```python
from build123d import *

# Parameters (mm, degrees)
SKETCH_1_W      = 90.450741223
SKETCH_1_H      = 43.255156446
EXTRUDE_1_DEPTH = 10
EXTRUDE_2_DEPTH = 20
EXTRUDE_3_DEPTH = 10


with BuildPart() as part:
    # 草图1 → 凸台-拉伸1 (new body)
    with BuildSketch(Plane(origin=(0, 0, 0), x_dir=(1, 0, 0), z_dir=(0, 1, 0))):
        with Locations((45.225370612, 21.627578223)):
            Rectangle(SKETCH_1_W, SKETCH_1_H)
    extrude(amount=EXTRUDE_1_DEPTH)

    # 草图2 → 凸台-拉伸2 (add)
    with BuildSketch(Plane(origin=(0, 10, 0), x_dir=(1, 0, 0), z_dir=(0, 1, 0))):
        with BuildLine():
            Line((68.630258788, 43.255156446), (21.047365446, 43.255156446))
            ThreePointArc((21.047365446, 43.255156446), (44.838812117, 19.463709775), (68.630258788, 43.255156446))
        make_face()
    extrude(amount=EXTRUDE_2_DEPTH)

    # 草图3 → 凸台-拉伸3 (add)
    with BuildSketch(Plane.XZ):
        with BuildLine():
            Line((22.99825717, -8.71008186), (70.802657673, -8.71008186))
            ThreePointArc((70.802657673, -8.71008186), (82.399412512, -20.3068367), (70.802657673, -31.903591539))
            Line((70.802657673, -31.903591539), (22.99825717, -31.903591539))
            ThreePointArc((22.99825717, -31.903591539), (11.40150233, -20.3068367), (22.99825717, -8.71008186))
        make_face()
    extrude(amount=EXTRUDE_3_DEPTH)


solid = part.part
```
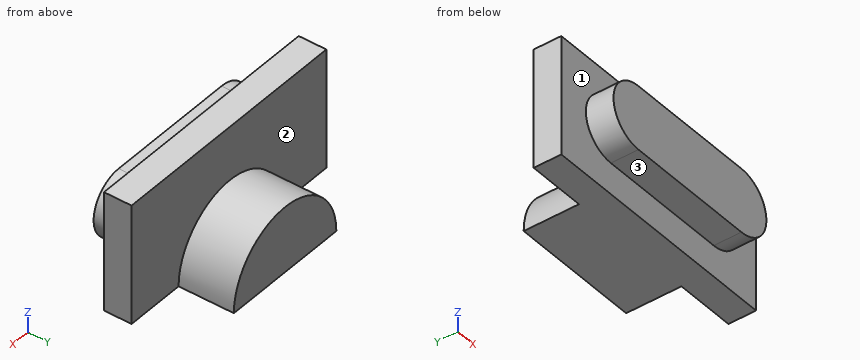
Read the model definition and answer for the solid it produces. Units are mm, in the model's axes. Face numbers are marked on the shaded views. A direction names the side the tool comes from. Coordinates: 2 decimals unless noted, no trailing zeros. Order: outer loops, then holes, each group sorted by start corner. A loop starts at its lowest first (then second) coordinate and runs counter-clockwise, first axis right, second up. Notation, with made-up numbers: (-15, 78) - (3, 78) arc R15 ccw to (3, 92) - close; hole circle Ø7 at (-13, 30). An arc over 180 degrees is marked (long way). Answer as a JSON object with one key per item and string values. Group by question number.
Item 1: Section B-B (z = -30.5) is taken. Give the vertices of the cut face in (x, y).
Item 2: Section A-A (x = 81.5) is taken. Give the vertices of the cut face in (y, z).
Item 3: Section D-D (x = 37.5) is taken. Give the vertices of the cut face in (y, z).
Item 4: Flat-ended cylindrical pins translate along their axes: P1, Ø10, axis at y = 22.5, z = -28.5, coming from the +X side; P2, Ø8, axis at x = 51, y = -5, coming from the -Z side; P3, Ø5, axis at x = 41.5, y = -4, coming from the +Z side. Find the tip coordinate at first contact, or state that the pin passes through.
Item 5: Consider probe 1 along Y at (x, z) = (73.5, -26); probe 2 along Z at (x, y) = (27.5, -1.5); probe 3 along Y at (x, z) = (76.5, -7). Determine where each line is inside the solid, lowest interval first. Write a range as from..to.
Item 6: A tool of negligible diameter and unlimited length cuts with its end or side. For the marked faces 1, 2 and 3, from which of +Z, -Z, +X, -X, +Y, -Y can it reach the whole face along a straight path? Write none if from no direction.
Results are:
{
 "1": {"outline": "(0, 0) - (17.47, 0) - (17.47, -10) - (76.33, -10) - (76.33, 0) - (90.45, 0) - (90.45, 10) - (64.92, 10) - (64.92, 30) - (24.76, 30) - (24.76, 10) - (0, 10) - close"},
 "2": {"outline": "(-10, -24.78) - (0, -24.78) - (0, -43.26) - (10, -43.26) - (10, 0) - (0, 0) - (0, -15.83) - (-10, -15.83) - close"},
 "3": {"outline": "(-10, -31.9) - (0, -31.9) - (0, -43.26) - (30, -43.26) - (30, -20.62) - (10, -20.62) - (10, 0) - (0, 0) - (0, -8.71) - (-10, -8.71) - close"},
 "4": {"P1": "stops at x = 66.54", "P2": "stops at z = -31.9", "P3": "stops at z = -8.71"},
 "5": {"probe 1": "y = -10..10", "probe 2": "z = -31.9..-8.71", "probe 3": "y = 0..10"},
 "6": {"face 1": "-Y", "face 2": "+Z, +Y", "face 3": "-Z, +X, -X, -Y"}
}
